```python
from build123d import *

# Parameters (mm, degrees)
ESQUISSE1_W        = 15
ESQUISSE1_H        = 11
BOSS_EXTRU_1_DEPTH = 4
CHANFREIN1_SIZE    = 1
ESQUISSE2_W        = 11
ESQUISSE2_H        = 7
BOSS_EXTRU_2_DEPTH = 8
CHANFREIN3_SIZE    = 1


with BuildPart() as part:
    # Esquisse1 → Boss.-Extru.1 (new body)
    with BuildSketch(Plane(origin=(0, 0, 0), x_dir=(1, 0, 0), z_dir=(0, 1, 0))):
        Rectangle(ESQUISSE1_W, ESQUISSE1_H)
    extrude(amount=-BOSS_EXTRU_1_DEPTH)

    # Chanfrein1
    chanfrein1_edges = [part.edges().sort_by_distance(p)[0] for p in [
        (7.5, -2, 5.5),
        (-7.5, -2, 5.5),
        (-7.5, -2, -5.5),
        (7.5, -2, -5.5),
    ]]
    chamfer(chanfrein1_edges, length=CHANFREIN1_SIZE)

    # Esquisse2 → Boss.-Extru.2 (add)
    with BuildSketch(Plane(origin=(0, 0, 0), x_dir=(1, 0, 0), z_dir=(0, 1, 0))):
        Rectangle(ESQUISSE2_W, ESQUISSE2_H)
    extrude(amount=BOSS_EXTRU_2_DEPTH)

    # Chanfrein3
    chanfrein3_edges = [part.edges().sort_by_distance(p)[0] for p in [
        (5.5, 4, 3.5),
        (5.5, 4, -3.5),
        (-5.5, 4, -3.5),
        (-5.5, 4, 3.5),
    ]]
    chamfer(chanfrein3_edges, length=CHANFREIN3_SIZE)


solid = part.part
```
Can you work these out from the model? Positions are in its coordinate system, mm. A direction names the side the tool comes from. Round coordinates to 2 decimals unless told otherwise and drop trailing zeros. Loops run counter-clockwise (first coordinate to the right, second up) from the corner with the lowest first, then second, coordinate; pieces in that order, holes last.
Item 1: Will these pins go through, and if not, where does the flat tip stop? pin 1 Ø6.5 at (x, y) = (-0.5, 6) entering from +Z; pin 2 Ø6.5 at (x, y) = (-2, 5.5) entering from -Z; pin 3 Ø2.5 at (y, z) = (4.5, -1) entering from +X.
Item 2: Suppose I cut it at C-C, the plane z = 4.75. Write out the boundary of the cut face in (x, y), then the cut area to 3 significant figures.
Item 3: Suppose I cut it at A-A, the plane z = 3. Write out the boundary of the cut face in (x, y).
Item 4: Please list where these lines run through material, in increasing order: L1, parallel to Y at x = -3.5, z = -4; L2, parallel to Z at x = -1, y = 1; L3, parallel to X at y = 2, z = 1.25.
Item 5: Which directions (+Z, -Z, +X, -X, +Y, -Y) give clear straight access to the entire face, cutting with the end or side of a thin tool? Please do faces 1 (the flat face through (-5, 4, -3)), 2 (the flat face through (0, 4, -3.5)), 3 (the flat face through (5, 4, 3)).
Item 6: Suppose I cut it at D-D, the plane z = -3.75. Write out the boundary of the cut face in (x, y), then the cut area to 3 significant figures.
Item 7: Suppose I cut it at B-B, the plane y = 5.5. Write out the boundary of the cut face in (x, z).
Reported:
1. pin 1: stops at z = 3.5
1. pin 2: stops at z = -3.5
1. pin 3: stops at x = 5.5
2. outline: (-7.25, -4) - (7.25, -4) - (7.25, 0) - (-7.25, 0) - close
2. area: 58.0 mm2
3. outline: (-7.5, -4) - (7.5, -4) - (7.5, 0) - (5, 0) - (5, 8) - (-5, 8) - (-5, 0) - (-7.5, 0) - close
4. L1: y = -4 to 0
4. L2: z = -3.5 to 3.5
4. L3: x = -5.5 to 5.5
5. face 1: -Z, -X, +Y
5. face 2: -Z, +X, -X, +Y
5. face 3: +Z, +X, +Y
6. outline: (-7.5, -4) - (7.5, -4) - (7.5, 0) - (-7.5, 0) - close
6. area: 60.0 mm2
7. outline: (-5.5, -2.5) - (-4.5, -3.5) - (4.5, -3.5) - (5.5, -2.5) - (5.5, 2.5) - (4.5, 3.5) - (-4.5, 3.5) - (-5.5, 2.5) - close
